Autodesk Inventor part; units mm, degrees
ref_plane "YZ Plane" through (0, 0, 0) normal (1, 0, 0) x (0, 1, 0)
ref_plane "XZ Plane" through (0, 0, 0) normal (0, 1, 0) x (-1, 0, 0)
ref_plane "XY Plane" through (0, 0, 0) normal (0, 0, 1) x (1, 0, 0)
sketch "Sketch1" plane through (0, 0, 0) normal (0, 1, 0) x (-1, 0, 0)
  circle A0 centre (0, 0) radius 7.5
  circle A1 centre (0, 0) radius 10
  dimension "d0" = 15
  dimension "d1" = 20
extrude "Extrusion1" add sketch "Sketch1" along normal blind 3
sketch "Sketch2" plane through (0, 3, 0) normal (0, 1, 0) x (1, 0, 0)
  circle A0 centre (0, 0) radius 9.6429
  circle A1 centre (0, 0) radius 13.5
  circle A2 centre (0, 0) radius 7.5
  dimension "d4" = 27
extrude "Extrusion2" add sketch "Sketch2" against normal up to surface (3 mm away) contours A0 | A1 | A2
sketch "Sketch3" plane through (0, 0, 0) normal (0, -1, 0) x (1, 0, 0)
  circle A0 centre (0, 0) radius 7.5
  dimension "d7" = 15
extrude "Extrusion3" cut sketch "Sketch3" against normal up to surface (3 mm away)
sketch "Sketch4" plane through (0, 3, 0) normal (0, 1, 0) x (1, 0, 0)
  circle A0 centre (0, 0) radius 12
  circle A1 centre (0, 0) radius 13.5
  dimension "d10" = 24
extrude "Extrusion4" cut sketch "Sketch4" against normal up to surface (3 mm away)
properties part number "DedoSoporte"
Geometry check sheet. Reference: the model listing, model coordinates, mm. Round coordinates to 2 decimals unless told otherwise and drop trailing zeros. Order: outer loops, then holes, each group sorted by start corner. A loop starts at its lowest first (then second) coordinate and runs counter-clockwise, first axis right, second up. Notation, with made-up numbers: M 14,31 L 39,31 A17 cw 39,55 Z; hole C 24,-29.75 d5. An arc over 180 degrees is marked long. Answer in a Markdown table with one row per item.
(1) Scan lines: probe 1 along Z at (x, y) = (0, 1.1); probe 2 along X at (y, z) = (1.9, -1.5); probe 3 along X at (y, z) = (0.65, 6). Record each from-to range of solid material in increasing order. Write a range as from..to.
Responses:
| item | result |
|---|---|
| probe 1 | z = -12..-7.5, 7.5..12 |
| probe 2 | x = -11.91..-7.35, 7.35..11.91 |
| probe 3 | x = -10.39..-4.5, 4.5..10.39 |
(2) Sectioned sample at B-B, the plane x = 0. Record the cut outline in (y, z).
Responses:
| item | result |
|---|---|
| outline | M 0,-12 L 3,-12 L 3,-7.5 L 0,-7.5 Z; M 0,7.5 L 3,7.5 L 3,12 L 0,12 Z |
(3) Draft check along X on faces 1 (the face through (-11.99, 1.52, -0.53)), 2 (the face through (-6, 0, 5)), 3 (the face through (-7.493, 1.479, 0.33)). Enter one of: released by +X, released by -X, zero draft, split by the parting line, or undercut.
Responses:
| item | result |
|---|---|
| face 1 | split by the parting line |
| face 2 | zero draft |
| face 3 | undercut |
(4) Sectioned sample at A-A, the plane z = 0. Record the cut outline in (x, y).
Responses:
| item | result |
|---|---|
| outline | M -12,0 L -7.5,0 L -7.5,3 L -12,3 Z; M 7.5,0 L 12,0 L 12,3 L 7.5,3 Z |
(5) Sectioned sample at C-C, the plane y = 1.95. Record the cut outline in (x, z), and give its area (3 significant figures).
Responses:
| item | result |
|---|---|
| outline | C 0,0 d24; hole C 0,0 d15 |
| area | 276 mm² |
(6) Sectioned sample at D-D, the plane x = -9.5. Record the cut outline in (y, z).
Responses:
| item | result |
|---|---|
| outline | M 0,-7.33 L 3,-7.33 L 3,7.33 L 0,7.33 Z |
